The listing builds one solid part. Answer for the finished solid, in the listing's coordinates (mm). A direction names the side the tool comes from. Round coordinates to 2 decimals unless told otherwise and drop trailing zeros. Write each loop counter-clockwise with the first axis right and the second up, starting at its lowest first coordinate (ties: lowest second). Pieces come first, ordered by that corner, then holes. Notation, with made-up numbers: (24.5, 20.25) - (58.5, 20.25) arc R37 ccw to (58.5, 58.25) - close; hole circle Ø2 at (36.5, -35). An arc over 180 degrees is marked (long way). Answer in a Markdown table with one row per item.
Autodesk Inventor part; units mm, degrees
ref_plane "YZ Plane" through (0, 0, 0) normal (1, 0, 0) x (0, 1, 0)
ref_plane "XZ Plane" through (0, 0, 0) normal (0, 1, 0) x (-1, 0, 0)
ref_plane "XY Plane" through (0, 0, 0) normal (0, 0, 1) x (1, 0, 0)
sketch "Эскиз1" plane through (0, 0, 0) normal (0, 0, 1) x (1, 0, 0)
  circle A0 centre (-9.5, 0) radius 7
  circle A1 centre (9.5, 0) radius 7
  line L0 (16.5, 0) -> (-16.5, 0)
  line L1 (9.5, -7) -> (-9.5, -7)
  line L2 (9.5, 7) -> (-9.5, 7)
  point P0 (0, 0)
  point P1 (0, 0)
  dimension "d0" = 14
  dimension "d1" = 14
  dimension "d2" = 33
extrude "Выдавливание1" add sketch "Эскиз1" along normal blind 5 and the other way blind 10
sketch "Эскиз2" plane through (0, 0, 5) normal (0, 0, 1) x (1, 0, 0)
  arc A0 (9.5, -7) -> (9.5, 7) centre (9.5, 0) ccw
  circle A1 centre (9.5, 0) radius 7
  arc A2 (-9.5, 7) -> (-9.5, -7) centre (-9.5, 0) ccw
  circle A3 centre (-9.5, 0) radius 7
  point P0 (0, 0)
  point P1 (-9.5, -7)
extrude "Выдавливание2" add sketch "Эскиз2" along normal blind 18
sketch "Эскиз3" plane through (0, 0, -10) normal (0, 0, -1) x (-1, 0, 0)
  arc A0 (9.5, -7) -> (9.5, 7) centre (9.5, 0) ccw
  circle A1 centre (9.5, 0) radius 5
  arc A2 (-9.5, 7) -> (-9.5, -7) centre (-9.5, 0) ccw
  circle A3 centre (-9.5, 0) radius 5
  point P0 (0, 0)
  dimension "d9" = 10
  dimension "d10" = 10
extrude "Выдавливание3" add sketch "Эскиз3" along normal blind 12
ref_plane "РабПлоскость1" through (-90.9653, 8.5, 0) normal (0, 0, 1) x (1, 0, 0)
sketch "Эскиз4" plane through (-90.9653, 8.5, 0) normal (0, 0, 1) x (1, 0, 0)
  circle A0 centre (100.4653, -8.5) radius 7
  circle A1 centre (81.4653, -8.5) radius 7
  arc A2 (100.4653, -15.5) -> (100.4653, -1.5) centre (100.4653, -8.5) ccw
  arc A3 (81.4653, -1.5) -> (81.4653, -15.5) centre (81.4653, -8.5) ccw
  line L0 (100.4653, -8.5) -> (81.4653, -8.5)
  line L1 (90.9653, -8.5) -> (90.9653, 7)
  line L2 (90.9653, -8.5) -> (70, -8.5)
properties part number "banana plug"
(1) For faces 1 (the cylindrical face through (4.73, -1.5, -15.92)), 2 (the cylindrical face through (-16.493, -0.308, 9.936)), 3 (the flat face through (10, 0, -22)), determine the directions among +Z, -Z, +X, -X, +Y, -Y from which every point of the face is accessible in a straight line to the end or side of a thin tool.
Checked values:
| item | result |
|---|---|
| face 1 | -Z |
| face 2 | +Z |
| face 3 | -Z, +X, -X, +Y, -Y |
(2) Section D-D (z = 1.5) is taken. Give the vertices of the cut face in (x, y), and give its area (3 significant figures).
Checked values:
| item | result |
|---|---|
| outline | (-9.5, -7) - (9.5, -7) arc R7 ccw to (9.5, 7) - (-9.5, 7) arc R7 ccw to start |
| area | 420 mm2 |
(3) Section A-A (z = -18) is taken. Give the vertices of the cut face in (x, y).
Checked values:
| item | result |
|---|---|
| outline | circle Ø10 at (-9.5, 0); circle Ø10 at (9.5, 0) |
(4) Section C-C (x = -10) is taken. Give the vertices of the cut face in (y, z).
Checked values:
| item | result |
|---|---|
| outline | (-6.98, -10) - (-4.97, -10) - (-4.97, -22) - (4.97, -22) - (4.97, -10) - (6.98, -10) - (6.98, 23) - (-6.98, 23) - close |
(5) Find the intervals of material crossed by line 1 (X direction, y = 0, z = 20.5); line 2 (Z direction, x = -3, y = -3.25); line 3 (X direction, y = 4.25, z = -17.5), in increasing order.
Checked values:
| item | result |
|---|---|
| line 1 | x = -16.5 to -2.5, 2.5 to 16.5 |
| line 2 | z = -10 to 5 |
| line 3 | x = -12.13 to -6.87, 6.87 to 12.13 |
(6) Flat-ended cylindrical pins translate along their axes: pin 1 (3 mm diameter, centred on y = 3, z = -3, fed in from -X); pin 2 (4 mm diameter, centred on y = -2.5, z = -7, fed in from +X); pin 3 (8 mm diameter, centred on y = -0.5, z = -0.5, fed in from -X); pin 4 (2 mm diameter, centred on x = -3, y = -2.5, fed in from -Z). Find the tip coordinate at first contact, or state that the pin passes through.
Checked values:
| item | result |
|---|---|
| pin 1 | stops at x = -16.34 |
| pin 2 | stops at x = 16.48 |
| pin 3 | stops at x = -16.5 |
| pin 4 | stops at z = -10 |
(7) Section B-B (y = 0) is taken. Give the vertices of the cut face in (x, z).
Checked values:
| item | result |
|---|---|
| outline | (-16.5, -10) - (-14.5, -10) - (-14.5, -22) - (-4.5, -22) - (-4.5, -10) - (4.5, -10) - (4.5, -22) - (14.5, -22) - (14.5, -10) - (16.5, -10) - (16.5, 23) - (2.5, 23) - (2.5, 5) - (-2.5, 5) - (-2.5, 23) - (-16.5, 23) - close |
(8) For a pull along X with two mould halves and no side action, classify faces 4 (the flat face through (0, 7, -3)), 5 (the flat face through (0, 0, -10)) as pulls with the +X half, pulls with the -X half, needs draft (parallel to the pull), parting line crosses it, or undercut.
Checked values:
| item | result |
|---|---|
| face 4 | needs draft |
| face 5 | undercut |
